from build123d import *

# Parameters (mm, degrees)
F0_W          = 40
F0_H          = 40
F1_DEPTH      = 20
F1_DEPTH_BACK = 20
F3_D          = 11
F4_R          = 10


with BuildPart() as f1:
    # F0 (on Top) → F1 (new body, two sides)
    with BuildSketch(Plane.XY) as f1_sk:
        Rectangle(F0_W, F0_H)
    extrude(amount=F1_DEPTH)
    extrude(f1_sk.sketch, amount=-F1_DEPTH_BACK)

    # F3 (through all)
    with Locations(Plane.XY.offset(20)):
        with Locations((0, 0)):
            Hole(F3_D / 2)

    # F4
    f4_edges = [f1.edges().sort_by_distance(p)[0] for p in [
        (0, -20, -20),
        (20, -20, 0),
        (-20, -20, 0),
        (0, -20, 20),
    ]]
    fillet(f4_edges, radius=F4_R)


solid = f1.part
Geometry: final body of the model. Coordinates: model frame, mm. Give positions to 0.01 mm unless a question says otherwise; leave off trailing zeros. Order: outer loops, then holes, each group sorted by start corner. A loop starts at its lowest first (then second) coordinate and runs counter-clockwise, first axis right, second up. Notation, with made-up numbers: (43.5, -24) -> (91.5, -24) arc R20 ccw to (91.5, -7) -> close; hole circle Ø10 at (52, 58.25). An arc over 180 degrees is marked (long way). Put each result on its own line as item: value.
Q1. Section C-C, the plane y = 0. Return loops of the section in (x, z).
Here are the results:
outline: (-20, -20) -> (-5.5, -20) -> (-5.5, 20) -> (-20, 20) -> close; (5.5, -20) -> (20, -20) -> (20, 20) -> (5.5, 20) -> close
Q2. Section B-B, the plane x = 0. Return loops of the section in (y, z).
Here are the results:
outline: (-20, -10) arc R10 ccw to (-10, -20) -> (-5.5, -20) -> (-5.5, 20) -> (-10, 20) arc R10 ccw to (-20, 10) -> close; (5.5, -20) -> (20, -20) -> (20, 20) -> (5.5, 20) -> close
Q3. Draft query along Y for faces 1 (the face through (1.19, -5.37, -0.28)), 2 (the face through (0, 20, 0)), 3 (the face through (0, 9, -20)), 4 (the face through (-18, -16, 0)). Return one class per face: released by +Y, released by -Y, zero draft, split by the parting line, or undercut.
Here are the results:
face 1: undercut
face 2: released by +Y
face 3: zero draft
face 4: released by -Y
Q4. Section A-A, the plane z = -8.5. Return loops of the section in (x, y).
Here are the results:
outline: (-20, -10) arc R10 ccw to (-10, -20) -> (10, -20) arc R10 ccw to (20, -10) -> (20, 20) -> (-20, 20) -> close; hole circle Ø11 at (0, 0)
Q5. Material intervals for L1, parallel to Y at x = 0, z = 9; L2, parallel to Y at x = 0, z = 12; L3, parallel to X at y = 2.5, z = 2, sorted ascending.
Here are the results:
L1: y = -20 to -5.5, 5.5 to 20
L2: y = -19.8 to -5.5, 5.5 to 20
L3: x = -20 to -4.9, 4.9 to 20
Q6. Section D-D, the plane x = 9. Return loops of the section in (y, z).
Here are the results:
outline: (-20, -10) arc R10 ccw to (-10, -20) -> (20, -20) -> (20, 20) -> (-10, 20) arc R10 ccw to (-20, 10) -> close
Q7. Pin query (flat end, axial travel): pin 1 (1.5 mm diameter, centred on x = 11.5, z = 10, fed in from -Y); pin 2 (17.5 mm diameter, centred on x = 0, y = 0, fed in from +Z); pin 3 (5 mm diameter, centred on x = 7.5, z = 14.5, fed in from -Y). Return the tip coordinate at first contact, or that it passes through.
Here are the results:
pin 1: stops at y = -19.97
pin 2: stops at z = 20
pin 3: stops at y = -19.8
